Can you work these out from the model? Positions are in its coordinate system, mm. Face numbers are marked on the shaded views. Give positions to 0.01 mm unless a question says otherwise; leave off trailing zeros. Loops run counter-clockwise (first coordinate to the right, second up) from the corner with the lowest first, then second, coordinate; pieces in that order, holes last. Notation, with made-up numbers: (31.5, 70) - (49.5, 70) arc R14 ccw to (49.5, 89) - close; hole circle Ø6 at (-36, 62.25). An arc over 180 degrees is marked (long way). Answer as a JSON object with one key per item and string values. Group by question number.
Item 1: Please list where these lines run through material, in increasing order: L1, parallel to Y at x = -18, z = 1.5 (3 decimals); L2, parallel to X at y = -4, z = 4; L3, parallel to Y at x = 22.5, z = -4.5 (3 decimals).
Item 2: Thinking about a two-plate mould opening in Y: for the marked faces 1, 2, 3 and 4, which applies, pulls with the +Y half, pulls with the -Y half, needs draft (parallel to the pull), parting line crosses it, or undercut?
Item 3: Suppose I cut it at D-D on x = -23.5. Write out the boundary of the cut face in (y, z), and give its area (3 significant figures).
Item 4: Suppose I cut it at A-A on x = 1.51. Write out the boundary of the cut face in (y, z) (3 decimals).
Item 5: Suppose I cut it at B-B on y = -1.5. Write out the boundary of the cut face in (x, z).
Item 6: Suppose I cut it at C-C on z = -4. Write out the boundary of the cut face in (x, y) (3 decimals), and give its area (3 significant figures).
from build123d import *

# Parameters (mm, degrees)
BOSS_EXTRUDE1_DEPTH   = 6
M6X1_0_TAPPED_HOLE1_D = 5
M6_CLEARANCE_HOLE1_D  = 6.6


with BuildPart() as part:
    # Sketch2 → Boss-Extrude1 (new, symmetric)
    with BuildSketch(Plane.XY):
        Polygon((31.75, -15.875), (-19.75, -15.875), (-31.75, -6), (-31.75, 6), (-19.75, 15.875), (19.75, 15.875), (31.75, 3.875), align=None)
    extrude(amount=BOSS_EXTRUDE1_DEPTH, both=True)

    # M6x1.0 Tapped Hole1 (through all)
    with Locations(Plane(origin=(0, 0, -6), x_dir=(-1, 0, 0), z_dir=(0, 0, -1))):
        with Locations((17.75, 1.875), (-1.51, 1.875)):
            Hole(M6X1_0_TAPPED_HOLE1_D / 2)

    # M6 Clearance Hole1 (through all)
    with Locations(Plane(origin=(0, 0, -6), x_dir=(-1, 0, 0), z_dir=(0, 0, -1))):
        with Locations((-19.74843928, -4.125)):
            Hole(M6_CLEARANCE_HOLE1_D / 2)


solid = part.part
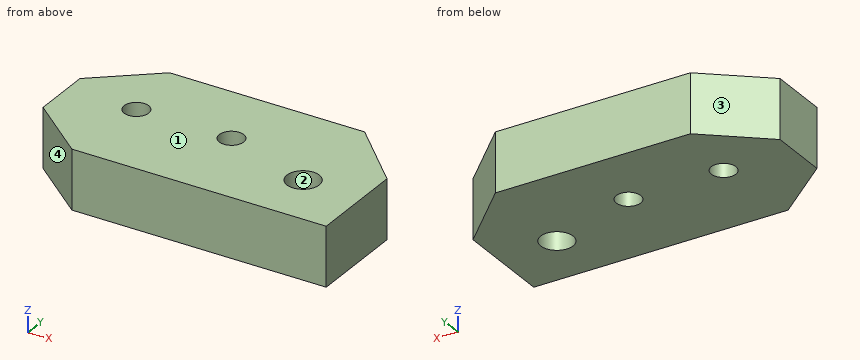
Worked out:
{
 "1": {"L1": "y = -15.875 to -0.612, 4.362 to 15.875", "L2": "x = -31.75 to 16.45, 23.05 to 31.75", "L3": "y = -15.875 to -5.947, -2.303 to 13.125"},
 "2": {"face 1": "needs draft", "face 2": "undercut", "face 3": "pulls with the +Y half", "face 4": "pulls with the -Y half"},
 "3": {"outline": "(-12.79, -6) - (12.79, -6) - (12.79, 6) - (-12.79, 6) - close", "area": "307 mm2"},
 "4": {"outline": "(-15.875, -6) - (-0.625, -6) - (-0.625, 6) - (-15.875, 6) - close; (4.375, -6) - (15.875, -6) - (15.875, 6) - (4.375, 6) - close"},
 "5": {"outline": "(-31.75, -6) - (17.75, -6) - (17.75, 6) - (-31.75, 6) - close; (21.75, -6) - (31.75, -6) - (31.75, 6) - (21.75, 6) - close"},
 "6": {"outline": "(-31.75, -6) - (-19.75, -15.875) - (31.75, -15.875) - (31.75, 3.875) - (19.75, 15.875) - (-19.75, 15.875) - (-31.75, 6) - close; hole circle Ø5 at (-17.75, 1.875); hole circle Ø5 at (1.51, 1.875); hole circle Ø6.6 at (19.748, -4.125)", "area": "1,750 mm2"}
}
